Study the drawing (mm; zero at the part's minimum x, y, z) and answer. Coordinates: 2 decimals unless noted, no trailing zeros. Write each loop counter-clockwise with the first axis right and the second up, starting at its lowest first coordinate (ties: lowest second). Pieces come first, ordered by that corner, then holes. Notation, with made-up numbers: (-24, 56) -> (27, 56) arc R31 cw to (27, 86) -> close; hole circle Ø10 at (85.5, 49). An arc over 180 degrees is marked (long way). Write item = value, one per line. Start each with the question number.
1) Section B-B (x = 12) is taken. Determine the outline of the cut face in (y, z), plus the area to 3 significant figures.
2) Section A-A (z = 19.05) is taken. Determine the outline of the cut face in (x, y), plus the area to 3 significant figures.
3) For a pull along Z with two mould halves and no side action, classify the marked faces 1, 2, 3 and 4 as released by +Z, released by -Z, zero draft, split by the parting line, or undercut.
4) Find the intervals of material crossed by line 1 along Z through (x, y) = (11, 12.75) (1 decimal); line 2 along X through (y, z) = (4.5, 24.5) (1 decimal); line 3 along X through (y, z) = (8.5, 15.5), in increasing order. Write a range as from..to.
5) Section C-C (x = 19.05) is taken. Determine the outline of the cut face in (y, z), plus the area to 3 significant figures.
6) Section D-D (y = 13.25) is taken. Count the separate pieces of the cut face and the enclosed holes in it, plus the area to 3 significant figures.
7) Flat-ended cylindrical pins translate along their axes: pin 1 Ø2.5 at (x, z) = (14.16, 14.16) entering from -Y; pin 2 Ø4 at (x, z) = (20.5, 20) entering from -Y; pin 3 Ø5 at (y, z) = (2.5, 22) entering from +X; pin 4 Ø5 at (y, z) = (8.5, 11) entering from -X. Find the tip coordinate at first contact, or state that the pin passes through.
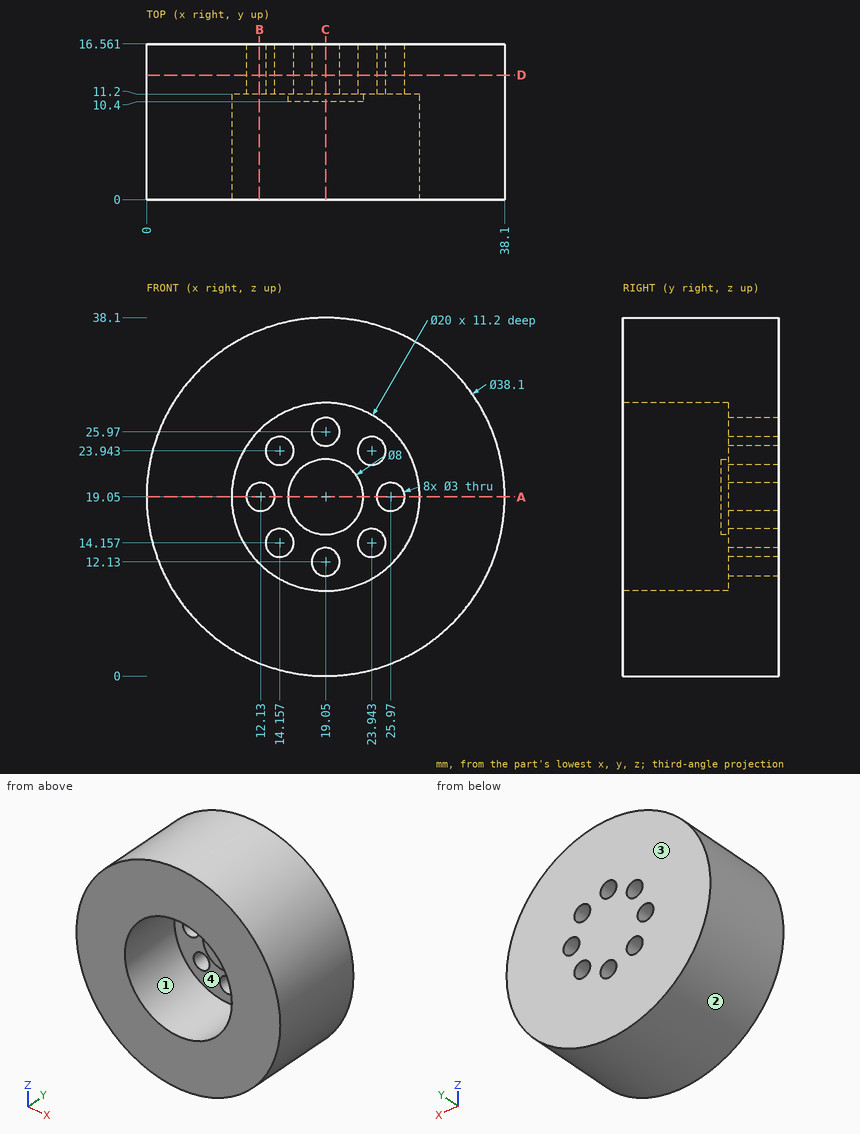
Answer key:
q1.outline = (0, 1.35) -> (16.56, 1.35) -> (16.56, 17.56) -> (11.2, 17.56) -> (11.2, 11.96) -> (0, 11.96) -> close; (0, 26.14) -> (11.2, 26.14) -> (11.2, 20.54) -> (16.56, 20.54) -> (16.56, 36.75) -> (0, 36.75) -> close
q1.area = 411 mm^2
q2.outline = (0, 0) -> (9.05, 0) -> (9.05, 11.2) -> (10.63, 11.2) -> (10.63, 16.56) -> (0, 16.56) -> close; (13.63, 11.2) -> (15.05, 11.2) -> (15.05, 10.4) -> (23.05, 10.4) -> (23.05, 11.2) -> (24.47, 11.2) -> (24.47, 16.56) -> (13.63, 16.56) -> close; (27.47, 11.2) -> (29.05, 11.2) -> (29.05, 0) -> (38.1, 0) -> (38.1, 16.56) -> (27.47, 16.56) -> close
q2.area = 381 mm^2
q3.face_1 = undercut
q3.face_2 = split by the parting line
q3.face_3 = zero draft
q3.face_4 = undercut
q4.line_1 = 1.8..18.1, 20..36.3
q4.line_2 = 0.8..10.7, 27.4..37.3
q4.line_3 = 0.33..9.7, 28.4..37.77
q5.outline = (0, 0) -> (16.56, 0) -> (16.56, 10.63) -> (11.2, 10.63) -> (11.2, 9.05) -> (0, 9.05) -> close; (0, 29.05) -> (11.2, 29.05) -> (11.2, 27.47) -> (16.56, 27.47) -> (16.56, 38.1) -> (0, 38.1) -> close; (10.4, 15.05) -> (11.2, 15.05) -> (11.2, 13.63) -> (16.56, 13.63) -> (16.56, 24.47) -> (11.2, 24.47) -> (11.2, 23.05) -> (10.4, 23.05) -> close
q5.area = 381 mm^2
q6.separate_pieces = 1
q6.enclosed_holes = 8
q6.area = 1,080 mm^2
q7.pin_1 = through
q7.pin_2 = 10.4
q7.pin_3 = 38.09
q7.pin_4 = 0.83
